Source: three-view drawing plus pictorial views. Frame: mm from the lowest corner of the part. A direction names the side the tool comes from. Give positions to 0.01 mm unless a question says otherwise; leave off trailing zeros. Loops run counter-clockwise (first coordinate to the right, second up) from the corner with the lowest first, then second, coordinate; pieces in that order, holes last. Notation, with made-up numbers: (-33, -22.75) - (23, -22.75) arc R17 ccw to (23, -18.75) - close; hole circle Ø7 at (36.5, 15). An arc over 180 degrees is marked (long way). Put each result on its own line as item: value.
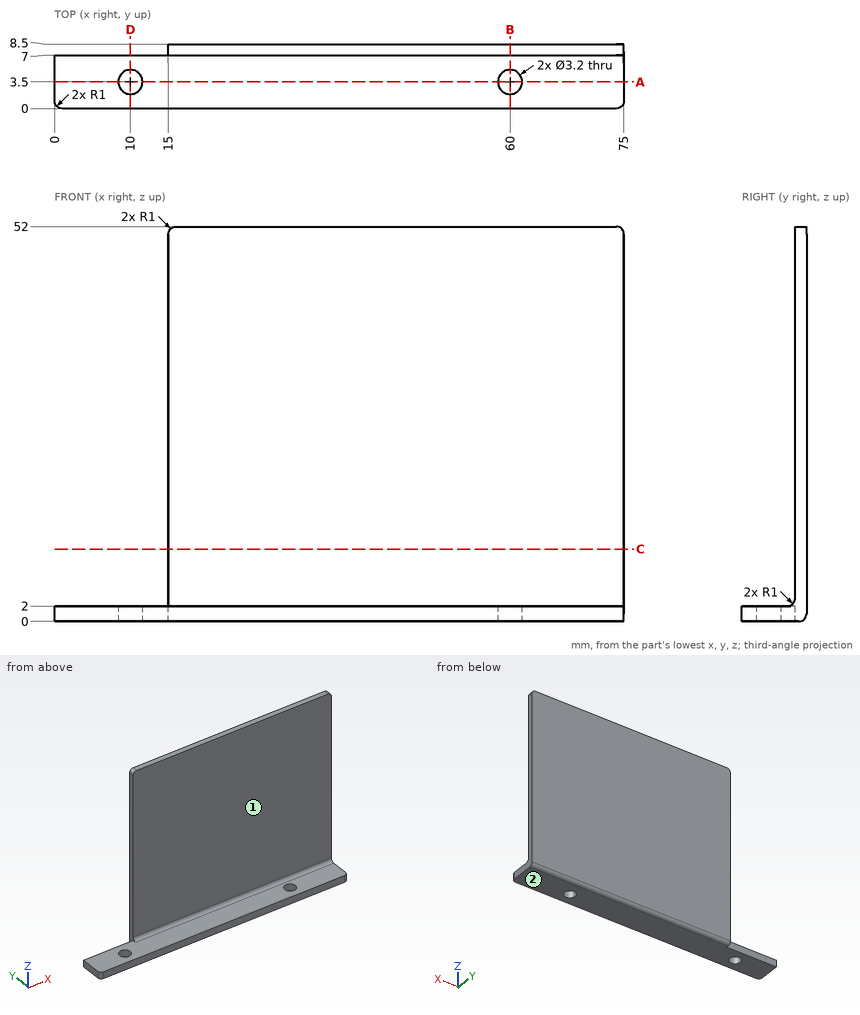
1) Section query B-B, the plane x = 60. Output: boundary loops of the cut face in (y, z), plus the area to 3 significant figures.
Check result:
outline: (0, 0) - (1.9, 0) - (1.9, 2) - (0, 2) - close; (5.1, 0) - (7.5, 0) arc R1 ccw to (8.5, 1) - (8.5, 52) - (7, 52) - (7, 3) arc R1 cw to (6, 2) - (5.1, 2) - close
area: 85.6 mm²
2) Section query C-C, the plane z = 9.5. Output: boundary loops of the cut face in (x, y).
Check result:
outline: (15, 7) - (75, 7) - (75, 8.5) - (15, 8.5) - close
3) Material intervals for line 1 along Y through (x, z) = (60, 1.3); line 2 along Y through (x, z) = (60, 0.6); line 3 along Z through (x, y) = (40.5, 5.5), sorted ascending. Write a range as [from, to].
Check result:
line 1: [0, 1.9], [5.1, 8.5]
line 2: [0, 1.9], [5.1, 8.42]
line 3: [0, 2]
4) Section query D-D, the plane x = 10. Output: boundary loops of the cut face in (y, z), plus the area to 3 significant figures.
Check result:
outline: (0, 0) - (1.9, 0) - (1.9, 2) - (0, 2) - close; (5.1, 0) - (7, 0) - (7, 2) - (5.1, 2) - close
area: 7.60 mm²
5) Section query A-A, the plane y = 3.5. Output: boundary loops of the cut face in (x, z), plus the area to 3 significant figures.
Check result:
outline: (0, 0) - (8.4, 0) - (8.4, 2) - (0, 2) - close; (11.6, 0) - (58.4, 0) - (58.4, 2) - (11.6, 2) - close; (61.6, 0) - (75, 0) - (75, 2) - (61.6, 2) - close
area: 137 mm²
6) Access query for the marked faces 1 and 2. Directions: +Z, -Z, +X, -X, +Y, -Y. A direction counts if a zero-diameter tool reaches every point of the face in a straight line with its end or side. Return the directions, or none.
Check result:
face 1: +Z, +X, -X, -Y
face 2: -Z, +X, -X, +Y, -Y
7) Pin query (flat end, axial travel): P1, Ø5, axis at y = 3.5, z = 7, coming from the +X side (1 decimal); P2, Ø2, axis at x = 5.5, z = 1, coming from the +Y side; P3, Ø2, axis at x = 44, y = 3.5, coming from the +Z side; P4, Ø5, axis at x = 52.5, z = 24, coming from the -Y side. Return the tip coordinate at first contact, or that it passes through.
Check result:
P1: through
P2: y = 7
P3: z = 2
P4: y = 7
